Can you work these out from the model? Positions are in its coordinate system, mm. Face numbers are marked on the shaded views. A direction names the side the tool comes from. Round coordinates to 2 decimals unless told otherwise and drop trailing zeros. Loops run counter-clockwise (first coordinate to the right, second up) from the corner with the lowest first, then second, coordinate; pieces in that order, holes last. Notation, with made-up numbers: (0, 10.5) -> (48, 10.5) arc R36 cw to (48, 48.5) -> close; hole circle Ø3 at (-4, 13). An arc over 180 degrees is marked (long way). Answer as a JSON object with one key per item and string values.
Autodesk Inventor part; units mm, degrees
ref_plane "YZ Plane" through (0, 0, 0) normal (1, 0, 0) x (0, 1, 0)
ref_plane "XZ Plane" through (0, 0, 0) normal (0, 1, 0) x (-1, 0, 0)
ref_plane "XY Plane" through (0, 0, 0) normal (0, 0, 1) x (1, 0, 0)
sketch "Sketch1" plane through (0, 0, 0) normal (1, 0, 0) x (0, 1, 0)
  line L0 (-25, 30) -> (25, 30)
  line L1 (30, 25) -> (30, -25)
  line L2 (25, -30) -> (-25, -30)
  line L3 (-30, -25) -> (-30, 25)
  line L4 (-30, 30) -> (30, -30) construction
  line L5 (30, 30) -> (-30, -30) construction
  arc A0 (-25, 30) -> (-30, 25) centre (-25, 25) ccw
  arc A1 (-30, -25) -> (-25, -30) centre (-25, -25) ccw
  arc A2 (25, -30) -> (30, -25) centre (25, -25) ccw
  arc A3 (30, 25) -> (25, 30) centre (25, 25) ccw
  circle A4 centre (-20, 0) radius 3
  circle A5 centre (15, 15) radius 3
  circle A6 centre (15, -15) radius 3
  point P0 (0, 0)
  dimension "d0" = 60
  dimension "d1" = 60
  dimension "d6" = 5
  dimension "d7" = 6
  dimension "d10" = 15
  dimension "d11" = 30
  dimension "d12" = 15
  dimension "d13" = 6
  dimension "d14" = 35
extrude "Plate1" add sketch "Sketch1" along normal mid plane 5
sketch "Sketch2" plane through (2.5, 0, 0) normal (1, 0, 0) x (0, 0, -1)
  line L0 (-30, -30) -> (-10, -30)
  line L1 (-10, -30) -> (-10, 0)
  line L2 (-10, 0) -> (-30, 0)
  line L3 (-30, 0) -> (-30, -30)
  line L4 (30, -30) -> (10, -30)
  line L5 (10, -30) -> (10, 0)
  line L6 (10, 0) -> (30, 0)
  line L7 (30, 0) -> (30, -30)
  circle A0 centre (-15, 15) radius 3
  circle A1 centre (0, -20) radius 3
  line L8 (-30, -25) -> (-30, 25) construction
  point P0 (0, 0)
  dimension "d15" = 15
  dimension "d17" = 10
  dimension "d18" = 10
  dimension "d19" = 30
extrude "Cut1" cut sketch "Sketch2" against normal blind 5 contours L3 L2 L1 L0 | L4 L5 L6 L7
fillet "Corner Round1" radius 6 2 edges at (0, -30, 10) (0, -30, -10)
equation "\"d20\" = Thickness"
equation "\"d9\" = Thickness"
equation "\"BendRadius\" = Thickness"
equation "\"BendReliefWidth\" = Thickness"
equation "\"BendReliefDepth\" = 0.5 * Thickness"
equation "\"TransitionRadius\" = BendRadius"
equation "\"JacobiRadiusSize\" = BendRadius"
equation "\"GapSize\" = Thickness"
properties part number "HCMUTE-CDT23-BAT_CANG_BANG_TAI" material "Stainless Steel"
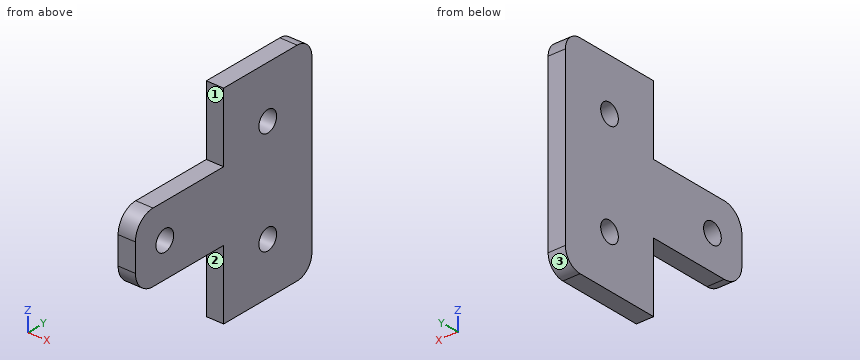
Q1. I want a section at D-D, the plane y = -20. Write out the boundary of the cut face in (x, z).
Determined:
{"outline": "(-2.5, -10) -> (2.5, -10) -> (2.5, -3) -> (-2.5, -3) -> close; (-2.5, 3) -> (2.5, 3) -> (2.5, 10) -> (-2.5, 10) -> close"}
Q2. I'm going to push flat-ended pins straight in: pin 1 (8 mm diameter, centred on y = 15, z = -15, fed in from +X); pin 2 (1.5 mm diameter, centred on x = -1, y = -15, fed in from -Z); pin 3 (1 mm diameter, centred on x = -1.5, z = -7, fed in from -Y); pin 4 (2.5 mm diameter, centred on x = -1, z = -24, fed in from -Y). Where does each tip first touch, or does it pass through?
Determined:
{"pin 1": "x = 2.5", "pin 2": "z = -10", "pin 3": "y = -29.45", "pin 4": "y = 0"}
Q3. I want a section at B-B, the plane y = 15. Write out the boundary of the cut face in (x, z), then the cut area to 3 significant figures.
Determined:
{"outline": "(-2.5, -30) -> (2.5, -30) -> (2.5, -18) -> (-2.5, -18) -> close; (-2.5, -12) -> (2.5, -12) -> (2.5, 12) -> (-2.5, 12) -> close; (-2.5, 18) -> (2.5, 18) -> (2.5, 30) -> (-2.5, 30) -> close", "area": "240 mm²"}
Q4. If I drill on L1, parallel to Z at x = 0.05, y = 15; L2, parallel to Z at x = 0.5, y = -20; L3, parallel to Z at x = -0.7, y = -22.5, over which ranges is the centre line in solid material (lowest first)? Write a range as [from, to].
Determined:
{"L1": "[-30, -18], [-12, 12], [18, 30]", "L2": "[-10, -3], [3, 10]", "L3": "[-10, -1.66], [1.66, 10]"}
Q5. I want a section at C-C, the plane x = -1.5. Write out the boundary of the cut face in (y, z), then the cut area to 3 significant figures.
Determined:
{"outline": "(-30, -4) arc R6 ccw to (-24, -10) -> (0, -10) -> (0, -30) -> (25, -30) arc R5 ccw to (30, -25) -> (30, 25) arc R5 ccw to (25, 30) -> (0, 30) -> (0, 10) -> (-24, 10) arc R6 ccw to (-30, 4) -> close; hole circle Ø6 at (-20, 0); hole circle Ø6 at (15, -15); hole circle Ø6 at (15, 15)", "area": "2,290 mm²"}
Q6. I want a section at A-A, the plane z = 15. Write out the boundary of the cut face in (x, y).
Determined:
{"outline": "(-2.5, 0) -> (2.5, 0) -> (2.5, 12) -> (-2.5, 12) -> close; (-2.5, 18) -> (2.5, 18) -> (2.5, 30) -> (-2.5, 30) -> close"}
Q7. On a 3-axis mill with a long thin cutter (end or side, diameter ignored), from which of +Z, -Z, +X, -X, +Y, -Y can I reach the whole of each face in a straight line? I mean the marked faces 1, 2 and 3. Say none if no direction works.
Determined:
{"face 1": "+Z, +X, -X, -Y", "face 2": "-Z, +X, -X, -Y", "face 3": "-Z, +X, -X, +Y"}
